from build123d import *

# Parameters (mm, degrees)
CHAMFER1_SIZE       = 0.5
CHAMFER1_SIZE2      = 1.866025404
CHAMFER2_SIZE       = 0.5
CHAMFER2_SIZE2      = 1.866025404
BOSS_EXTRUDE1_DEPTH = 7.4
SKETCH6_R           = 1.5
CUT_EXTRUDE1_DEPTH  = 10
CIRPATTERN1_COUNT   = 2
CIRPATTERN1_ANGLE   = 270


with BuildPart() as part:
    # Sketch2 → Revolve1 (revolve)
    with BuildSketch(Plane(origin=(0, 0, 0), x_dir=(0, 0, -1), z_dir=(1, 0, 0))):
        Polygon((-16, 2.5), (0, 2.5), (0, 8.9), (-7.6, 8.9), (-7.6, 6.1), (-15, 6.1), (-15, 8.9), (-16, 8.9), align=None)
    revolve(axis=Axis((0, 0, 79.609460318), (0, 0, -1)))

    # Chamfer1
    chamfer1_edges = [part.edges().sort_by_distance(p)[0] for p in [
        (0, -8.9, 15),
    ]]
    chamfer1_side = [part.faces().sort_by_distance(p)[0] for p in [
        (0, -8.9, 15.5),
    ]]
    chamfer(chamfer1_edges, length=CHAMFER1_SIZE, length2=CHAMFER1_SIZE2, reference=chamfer1_side[0])

    # Chamfer2
    chamfer2_edges = [part.edges().sort_by_distance(p)[0] for p in [
        (0, -8.9, 7.6),
    ]]
    chamfer2_side = [part.faces().sort_by_distance(p)[0] for p in [
        (0, -8.9, 3.8),
    ]]
    chamfer(chamfer2_edges, length=CHAMFER2_SIZE, length2=CHAMFER2_SIZE2, reference=chamfer2_side[0])

    # Sketch4 → Boss-Extrude1 (add)
    with BuildSketch(Plane.XY.offset(7.6)):
        with BuildLine():
            Line((1.645655792, 5.873824735), (1.892869388, 6.634669948))
            Line((1.892869388, 6.634669948), (2.368397646, 6.48016145))
            Line((2.368397646, 6.48016145), (2.121184051, 5.719316237))
            ThreePointArc((2.121184051, 5.719316237), (1.885003666, 5.801444749), (1.645655792, 5.873824735))
        make_face()
        with BuildLine():
            Line((-0.25, 6.094874896), (-0.25, 6.894874896))
            Line((-0.25, 6.894874896), (0.25, 6.894874896))
            Line((0.25, 6.894874896), (0.25, 6.094874896))
            ThreePointArc((0.25, 6.094874896), (0, 6.1), (-0.25, 6.094874896))
        make_face()
        with BuildLine():
            Line((3.38022333, 5.077803683), (3.850451532, 5.725017278))
            Line((3.850451532, 5.725017278), (4.254960029, 5.431124652))
            Line((4.254960029, 5.431124652), (3.784731827, 4.783911057))
            ThreePointArc((3.784731827, 4.783911057), (3.585490039, 4.935003666), (3.38022333, 5.077803683))
        make_face()
        with BuildLine():
            Line((4.783911057, 3.784731827), (5.431124652, 4.254960029))
            Line((5.431124652, 4.254960029), (5.725017278, 3.850451532))
            Line((5.725017278, 3.850451532), (5.077803683, 3.38022333))
            ThreePointArc((5.077803683, 3.38022333), (4.935003666, 3.585490039), (4.783911057, 3.784731827))
        make_face()
        with BuildLine():
            Line((5.719316237, 2.121184051), (6.48016145, 2.368397646))
            Line((6.48016145, 2.368397646), (6.634669948, 1.892869388))
            Line((6.634669948, 1.892869388), (5.873824735, 1.645655792))
            ThreePointArc((5.873824735, 1.645655792), (5.801444749, 1.885003666), (5.719316237, 2.121184051))
        make_face()
        with BuildLine():
            Line((6.094874896, 0.25), (6.894874896, 0.25))
            Line((6.894874896, 0.25), (6.894874896, -0.25))
            Line((6.894874896, -0.25), (6.094874896, -0.25))
            ThreePointArc((6.094874896, -0.25), (6.1, 0), (6.094874896, 0.25))
        make_face()
        with BuildLine():
            Line((5.873824735, -1.645655792), (6.634669948, -1.892869388))
            Line((6.634669948, -1.892869388), (6.48016145, -2.368397646))
            Line((6.48016145, -2.368397646), (5.719316237, -2.121184051))
            ThreePointArc((5.719316237, -2.121184051), (5.801444749, -1.885003666), (5.873824735, -1.645655792))
        make_face()
        with BuildLine():
            Line((5.077803683, -3.38022333), (5.725017278, -3.850451532))
            Line((5.725017278, -3.850451532), (5.431124652, -4.254960029))
            Line((5.431124652, -4.254960029), (4.783911057, -3.784731827))
            ThreePointArc((4.783911057, -3.784731827), (4.935003666, -3.585490039), (5.077803683, -3.38022333))
        make_face()
        with BuildLine():
            Line((3.784731827, -4.783911057), (4.254960029, -5.431124652))
            Line((4.254960029, -5.431124652), (3.850451532, -5.725017278))
            Line((3.850451532, -5.725017278), (3.38022333, -5.077803683))
            ThreePointArc((3.38022333, -5.077803683), (3.585490039, -4.935003666), (3.784731827, -4.783911057))
        make_face()
        with BuildLine():
            Line((2.121184051, -5.719316237), (2.368397646, -6.48016145))
            Line((2.368397646, -6.48016145), (1.892869388, -6.634669948))
            Line((1.892869388, -6.634669948), (1.645655792, -5.873824735))
            ThreePointArc((1.645655792, -5.873824735), (1.885003666, -5.801444749), (2.121184051, -5.719316237))
        make_face()
        with BuildLine():
            Line((0.25, -6.094874896), (0.25, -6.894874896))
            Line((0.25, -6.894874896), (-0.25, -6.894874896))
            Line((-0.25, -6.894874896), (-0.25, -6.094874896))
            ThreePointArc((-0.25, -6.094874896), (0, -6.1), (0.25, -6.094874896))
        make_face()
        with BuildLine():
            Line((-1.645655792, -5.873824735), (-1.892869388, -6.634669948))
            Line((-1.892869388, -6.634669948), (-2.368397646, -6.48016145))
            Line((-2.368397646, -6.48016145), (-2.121184051, -5.719316237))
            ThreePointArc((-2.121184051, -5.719316237), (-1.885003666, -5.801444749), (-1.645655792, -5.873824735))
        make_face()
        with BuildLine():
            Line((-3.38022333, -5.077803683), (-3.850451532, -5.725017278))
            Line((-3.850451532, -5.725017278), (-4.254960029, -5.431124652))
            Line((-4.254960029, -5.431124652), (-3.784731827, -4.783911057))
            ThreePointArc((-3.784731827, -4.783911057), (-3.585490039, -4.935003666), (-3.38022333, -5.077803683))
        make_face()
        with BuildLine():
            Line((-4.783911057, -3.784731827), (-5.431124652, -4.254960029))
            Line((-5.431124652, -4.254960029), (-5.725017278, -3.850451532))
            Line((-5.725017278, -3.850451532), (-5.077803683, -3.38022333))
            ThreePointArc((-5.077803683, -3.38022333), (-4.935003666, -3.585490039), (-4.783911057, -3.784731827))
        make_face()
        with BuildLine():
            Line((-5.719316237, -2.121184051), (-6.48016145, -2.368397646))
            Line((-6.48016145, -2.368397646), (-6.634669948, -1.892869388))
            Line((-6.634669948, -1.892869388), (-5.873824735, -1.645655792))
            ThreePointArc((-5.873824735, -1.645655792), (-5.801444749, -1.885003666), (-5.719316237, -2.121184051))
        make_face()
        with BuildLine():
            Line((-6.094874896, -0.25), (-6.894874896, -0.25))
            Line((-6.894874896, -0.25), (-6.894874896, 0.25))
            Line((-6.894874896, 0.25), (-6.094874896, 0.25))
            ThreePointArc((-6.094874896, 0.25), (-6.1, 0), (-6.094874896, -0.25))
        make_face()
        with BuildLine():
            Line((-5.873824735, 1.645655792), (-6.634669948, 1.892869388))
            Line((-6.634669948, 1.892869388), (-6.48016145, 2.368397646))
            Line((-6.48016145, 2.368397646), (-5.719316237, 2.121184051))
            ThreePointArc((-5.719316237, 2.121184051), (-5.801444749, 1.885003666), (-5.873824735, 1.645655792))
        make_face()
        with BuildLine():
            Line((-5.077803683, 3.38022333), (-5.725017278, 3.850451532))
            Line((-5.725017278, 3.850451532), (-5.431124652, 4.254960029))
            Line((-5.431124652, 4.254960029), (-4.783911057, 3.784731827))
            ThreePointArc((-4.783911057, 3.784731827), (-4.935003666, 3.585490039), (-5.077803683, 3.38022333))
        make_face()
        with BuildLine():
            Line((-3.784731827, 4.783911057), (-4.254960029, 5.431124652))
            Line((-4.254960029, 5.431124652), (-3.850451532, 5.725017278))
            Line((-3.850451532, 5.725017278), (-3.38022333, 5.077803683))
            ThreePointArc((-3.38022333, 5.077803683), (-3.585490039, 4.935003666), (-3.784731827, 4.783911057))
        make_face()
        with BuildLine():
            Line((-2.121184051, 5.719316237), (-2.368397646, 6.48016145))
            Line((-2.368397646, 6.48016145), (-1.892869388, 6.634669948))
            Line((-1.892869388, 6.634669948), (-1.645655792, 5.873824735))
            ThreePointArc((-1.645655792, 5.873824735), (-1.885003666, 5.801444749), (-2.121184051, 5.719316237))
        make_face()
    extrude(amount=BOSS_EXTRUDE1_DEPTH)

    # Sketch6 → Cut-Extrude1 (cut)
    with BuildSketch(Plane(origin=(0, 8.9, 0), x_dir=(-1, 0, 0), z_dir=(0, 1, 0))):
        with Locations((0, 3.55)):
            Circle(SKETCH6_R)
    cut_extrude1 = extrude(amount=-CUT_EXTRUDE1_DEPTH, mode=Mode.SUBTRACT)

    # CirPattern1: Cut-Extrude1 ×2 about axis
    cirpattern1_axis = Axis((0, 0, 0), (0, 0, 1))
    for i in range(1, CIRPATTERN1_COUNT):
        add(cut_extrude1.rotate(cirpattern1_axis, i * CIRPATTERN1_ANGLE / (CIRPATTERN1_COUNT - 1)), mode=Mode.SUBTRACT)


solid = part.part
The listing builds one solid part. Answer for the finished solid, in the listing's coordinates (mm). A direction names the side the tool comes from. Coordinates: 2 decimals unless noted, no trailing zeros. Loops run counter-clockwise (first coordinate to the right, second up) from the corner with the lowest first, then second, coordinate; pieces in that order, holes last. Notation, with made-up numbers: (5.5, 32) -> (41.5, 32) arc R24 ccw to (41.5, 64) -> close; hole circle Ø10 at (60.5, 26.25). An arc over 180 degrees is marked (long way). Write item = value, one per line. Start each with the question number.
1) A tool of negligible diameter and unlimited length cuts with its end or side. For faces 1 (the face through (-8.69, -1.93, 3.6)), 2 (the face through (6.026, -0.944, 11.352)), 3 (the face through (0.964, -6.023, 11.352)), 4 (the face through (5.44, -2.76, 11.35)), 5 (the face through (0.944, 6.026, 11.352)), from which of +Z, -Z, +X, -X, +Y, -Y can it reach the whole face along a straight path? Write none if from no direction.
2) A cutting plane is placed at C-C (z = 3.55). Give the vertices of the cut face in (x, y), then the cut area to 3 significant figures.
3) Given pin 1 Ø5 at (y, z) = (-6, 11.5) entering from -X (3 decimals); pin 2 Ø0.6 at (x, z) = (-6.5, 10) entering from +Y; pin 3 Ø0.9 at (y, z) = (6.5, 10) entering from +X, each flat-ended and moving along its own axis, determine where each tip first touches the part or whether it passes through.
4) Straight lines are drawn through the part: line 1 (X direction, y = 0, z = 9.5); line 2 (Y direction, x = -5.25, z = 7.75); line 3 (Z direction, x = 4.25, y = 0). For each, find the intervals that lie inside material, in ascending order. Write a range as from..to.
5) The mould has two halves that part along X. Classify faces 6 (the face through (-8.69, -1.93, 15.75)), 7 (the face through (4.306, 4.32, 11.352)), 8 (the face through (-6.023, -0.964, 11.352)): released by +X, released by -X, zero draft, split by the parting line, or undercut.
6) A cutting plane is placed at D-D (x = 8). Count the separate pieces of the cut face and the enclosed holes in it, then the cut area to 3 significant figures.
7) A cutting plane is placed at A-A (x = 0). Give the vertices of the cut face in (y, z), then the cut area to 3 significant figures.
Responses:
q1.face_1 = +Z, -Z
q1.face_2 = +X
q1.face_3 = -Y
q1.face_4 = none
q1.face_5 = +Y
q2.outline = (-1.5, 2) -> (-1.5, 8.77) arc R8.9 ccw (long way) to (8.77, -1.5) -> (2, -1.5) arc R2.5 cw (long way) to start; (1.5, 2) arc R2.5 cw to (2, 1.5) -> (8.77, 1.5) arc R8.9 ccw to (1.5, 8.77) -> close
q2.area = 190 mm²
q3.pin_1 = -5.725
q3.pin_2 = 2.37
q3.pin_3 = 2.37
q4.line_1 = -6.89..-2.5, 2.5..6.89
q4.line_2 = -4.12..-3.51, -3.11..3.11, 3.51..4.12
q4.line_3 = 0..2.05, 5.05..16
q5.face_6 = split by the parting line
q5.face_7 = undercut
q5.face_8 = released by -X
q6.separate_pieces = 2
q6.enclosed_holes = 1
q6.area = 54.7 mm²
q7.outline = (-8.9, 0) -> (-2.5, 0) -> (-2.5, 16) -> (-8.9, 16) -> (-8.9, 15.5) -> (-7.03, 15) -> (-6.89, 15) -> (-6.89, 7.6) -> (-7.03, 7.6) -> (-8.9, 7.1) -> close; (2.5, 0) -> (8.9, 0) -> (8.9, 2.05) -> (2.5, 2.05) -> close; (2.5, 5.05) -> (8.9, 5.05) -> (8.9, 7.1) -> (7.03, 7.6) -> (6.89, 7.6) -> (6.89, 15) -> (7.03, 15) -> (8.9, 15.5) -> (8.9, 16) -> (2.5, 16) -> close
q7.area = 154 mm²
